Verification items for the finished model (mm, model axes). Face numbers are marked on the shaded views. Coordinates: 2 decimals unless noted, no trailing zeros. Write each loop counter-clockwise with the first axis right and the second up, starting at its lowest first coordinate (ties: lowest second). Pieces come first, ordered by that corner, then holes. Notation, with made-up numbers: (79, 60) -> (108, 60) arc R8 ccw to (108, 64) -> close; hole circle Ø8 at (35.25, -8.75). An arc over 180 degrees is marked (long way). Use CSV: the item, a comma, the result in double quotes.
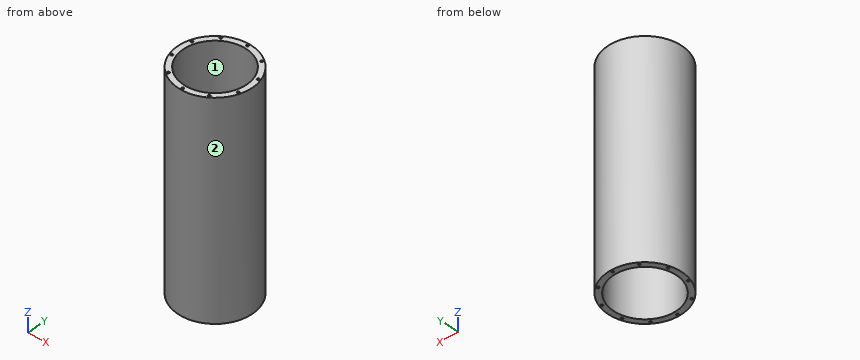
```python
from build123d import *

# Parameters (mm, degrees)
SKETCH_1_R               = 53
EXTRUDE_1_DEPTH          = 300
SKETCH_2_R               = 45
CUT_EXTRUDE_1_DEPTH      = 300
PATTERN_CIRCULAR_1_COUNT = 10
PATTERN_CIRCULAR_2_COUNT = 10


with BuildPart() as part:
    # Sketch 1 → Extrude 1 (new body)
    with BuildSketch(Plane.XY):
        Circle(SKETCH_1_R)
    extrude(amount=EXTRUDE_1_DEPTH)

    # Sketch 2 → Cut-Extrude 1 (cut)
    with BuildSketch(Plane(origin=(0, 0, 0), x_dir=(-1, 0, 0), z_dir=(0, 0, -1))):
        Circle(SKETCH_2_R)
    extrude(amount=-CUT_EXTRUDE_1_DEPTH, mode=Mode.SUBTRACT)

    # Sketch 3 → Hole Wizard M4 _1 (revolve, cut)
    with BuildSketch(Plane(origin=(0, 50, 0), x_dir=(0, 1, 0), z_dir=(1, 0, 0))):
        Polygon((0, 0), (0, 11.091420021), (1.65, 10.1), (1.65, 0), align=None)
    hole_wizard_m4_1 = revolve(axis=Axis((0, 50, -6.35), (0, 0, 1)), mode=Mode.SUBTRACT)

    # Pattern Circular 1: Hole Wizard M4 _1 ×10 about axis
    pattern_circular_1_axis = Axis((0, 0, 0), (0, 0, 1))
    for i in range(1, PATTERN_CIRCULAR_1_COUNT):
        add(hole_wizard_m4_1.rotate(pattern_circular_1_axis, i * 360 / PATTERN_CIRCULAR_1_COUNT), mode=Mode.SUBTRACT)

    # Sketch 5 → Hole Wizard M4 _2 (revolve, cut)
    with BuildSketch(Plane(origin=(0, 50, 300), x_dir=(0, -1, 0), z_dir=(1, 0, 0))):
        Polygon((0, 0), (0, 11.091420021), (1.65, 10.1), (1.65, 0), align=None)
    hole_wizard_m4_2 = revolve(axis=Axis((0, 50, 306.35), (0, 0, -1)), mode=Mode.SUBTRACT)

    # Pattern Circular 2: Hole Wizard M4 _2 ×10 about axis
    pattern_circular_2_axis = Axis((0, 0, 0), (0, 0, 1))
    for i in range(1, PATTERN_CIRCULAR_2_COUNT):
        add(hole_wizard_m4_2.rotate(pattern_circular_2_axis, i * 360 / PATTERN_CIRCULAR_2_COUNT), mode=Mode.SUBTRACT)


solid = part.part
```
1) Cross-section at A-A (y = 0). Record the boundary of the cut face in (x, z).
Return value:
outline,"(-53, 0) -> (-45, 0) -> (-45, 300) -> (-53, 300) -> close; (45, 0) -> (53, 0) -> (53, 300) -> (45, 300) -> close"
2) Scan lines: L1, parallel to Y at x = -2, z = 184; L2, parallel to X at y = 19, z = 65; L3, parallel to Y at x = 38, z = 117. Record each from-to range of solid material in increasing order.
Return value:
L1,"-52.96 to -44.96, 44.96 to 52.96"
L2,"-49.48 to -40.79, 40.79 to 49.48"
L3,"-36.95 to -24.1, 24.1 to 36.95"
3) Gauge pin test, flat ends, axial feed: pin 1 (4 mm diameter, centred on y = -31, z = 260.5, fed in from +X); pin 2 (2.5 mm diameter, centred on x = 47.55, y = -15.45, fed in from -Z); pin 3 (3 mm diameter, centred on x = -29.39, y = -40.45, fed in from +Z). Record the tip position at first contact, or that the pin passes through.
Return value:
pin 1,"x = 44.36"
pin 2,"z = 10.34"
pin 3,"z = 289.81"
4) Mould release check, pull along Y, two halves, no side actions. Record for the marked faces 1 and 2: released by +Y, released by -Y, zero draft, split by the parting line, or undercut.
Return value:
face 1,"undercut"
face 2,"split by the parting line"
5) Cross-section at C-C (z = 97.5). Record the boundary of the cut face in (x, y).
Return value:
outline,"circle Ø106 at (0, 0); hole circle Ø90 at (0, 0)"
6) Cross-section at B-B (x = -11). Record the boundary of the cut face in (y, z), plus the area to 3 significant figures.
Return value:
outline,"(-51.85, 0) -> (-43.63, 0) -> (-43.63, 300) -> (-51.85, 300) -> close; (43.63, 0) -> (51.85, 0) -> (51.85, 300) -> (43.63, 300) -> close"
area,"4,930 mm2"
